The listing builds one solid part. Answer for the finished solid, in the listing's coordinates (mm). A direction names the side the tool comes from. Round coordinates to 2 decimals unless told otherwise and drop trailing zeros. Write each loop counter-clockwise with the first axis right and the second up, starting at its lowest first coordinate (ties: lowest second). Pieces come first, ordered by that corner, then holes. Notation, with made-up numbers: (-38, -10.5) - (19, -10.5) arc R32 cw to (19, 27.5) - close; hole circle Ø6 at (-4.75, 75.25). An arc over 180 degrees is marked (long way). Answer as CSV lines item,"result". Start each with the question number.
Item 1: A cutting plane is placed at C-C on y = 42. Determine the outline of the cut face in (x, z).
Item 2: Flat-ended cylindrical pins translate along their axes: pin 1 (1.5 mm diameter, centred on x = 35, z = 1.5, fed in from -Y); pin 2 (6 mm diameter, centred on x = 25.5, y = 20, fed in from -Z); pin 3 (1.5 mm diameter, centred on x = 36.5, z = 3, fed in from +Y). Find the tip coordinate at first contact, or state that the pin passes through.
Item 3: A cutting plane is placed at D-D on z = 4. State how many separate pieces and enclosed holes the cut face has, and give its area (3 significant figures).
Item 4: A cutting plane is placed at A-A on y = 104.5. Determine the outline of the cut face in (x, z), and give its area (3 significant figures).
Item 5: A cutting plane is placed at B-B on x = 12. Determine the outline of the cut face in (y, z), and give its area (3 significant figures).
Item 6: For a pull along X with two mould halves and no side action, classify faces 4 (the flat face through (0, 96, 2)), 5 (the flat face through (12, 195, 2)), 6 (the flat face through (25, -3, 2)) as pulls with the +X half, pulls with the -X half, needs draft (parallel to the pull), parting line crosses it, or undercut.
Item 7: Which of the six approach directions +Z, -Z, +X, -X, +Y, -Y give full straight-line access (tool end or side, diameter ignored) to faces 1 (the flat face through (45, -3, 2)), 2 (the flat face through (35, 190, 2)), 3 (the flat face through (60, 51, 3))?
Item 8: Straight lines are drawn through the part: line 1 along Y through (x, z) = (31.5, 0.8); line 2 along Y through (x, z) = (47, 2.05); line 3 along X through (y, z) = (151, 1.75). For each, find the intervals that lie inside material, in ascending order. Write a range as [from, to].
```python
from build123d import *

# Parameters (mm, degrees)
SKETCH_1_W          = 25
SKETCH_1_H          = 5
SKETCH_1_W_2        = 70
SKETCH_1_H_2        = 190
EXTRUDE_1_DEPTH     = 5
SKETCH_2_R          = 1.55
CUT_EXTRUDE_1_DEPTH = 5
SKETCH_3_W          = 50
SKETCH_3_H          = 72.5
CUT_EXTRUDE_2_DEPTH = 5
FILLET_1_R          = 10
FILLET_2_R          = 1


with BuildPart() as part:
    # 草图1 → 凸台-拉伸1 (new body)
    with BuildSketch(Plane.XY):
        with Locations((57.5, 192.5)):
            Rectangle(SKETCH_1_W, SKETCH_1_H)
        with Locations((35, 95)):
            Rectangle(SKETCH_1_W_2, SKETCH_1_H_2)
        with Locations((12.5, 192.5)):
            Rectangle(SKETCH_1_W, SKETCH_1_H)
        with Locations((57.5, -2.5)):
            Rectangle(SKETCH_1_W, SKETCH_1_H)
        with Locations((12.5, -2.5)):
            Rectangle(SKETCH_1_W, SKETCH_1_H)
    extrude(amount=EXTRUDE_1_DEPTH)

    # 草图2 → 切除-拉伸1 (cut)
    with BuildSketch(Plane.XY.offset(5)):
        with Locations((43.45, 0)):
            Circle(SKETCH_2_R)
        with Locations((26.55, 0)):
            Circle(SKETCH_2_R)
        with Locations((43.45, 190)):
            Circle(SKETCH_2_R)
        with Locations((26.55, 190)):
            Circle(SKETCH_2_R)
    extrude(amount=-CUT_EXTRUDE_1_DEPTH, mode=Mode.SUBTRACT)

    # 草图3 → 切除-拉伸2 (cut)
    with BuildSketch(Plane.XY.offset(5)):
        with Locations((35, 51.25)):
            Rectangle(SKETCH_3_W, SKETCH_3_H)
        with Locations((35, 138.75)):
            Rectangle(SKETCH_3_W, SKETCH_3_H)
    extrude(amount=-CUT_EXTRUDE_2_DEPTH, mode=Mode.SUBTRACT)

    # 圆角1
    fillet_1_edges = [part.edges().sort_by_distance(p)[0] for p in [
        (10, 15, 2.5),
        (10, 87.5, 2.5),
        (60, 87.5, 2.5),
        (60, 15, 2.5),
        (10, 102.5, 2.5),
        (10, 175, 2.5),
        (60, 175, 2.5),
        (60, 102.5, 2.5),
    ]]
    fillet(fillet_1_edges, radius=FILLET_1_R)

    # 圆角2
    fillet_2_edges = [part.edges().sort_by_distance(p)[0] for p in [
        (45, 195, 2.5),
        (70, 195, 2.5),
        (70, -5, 2.5),
        (0, -5, 2.5),
        (0, 195, 2.5),
        (25, 195, 2.5),
    ]]
    fillet(fillet_2_edges, radius=FILLET_2_R)


solid = part.part
```
Geometry says:
1,outline,"(0, 0) - (10, 0) - (10, 5) - (0, 5) - close; (60, 0) - (70, 0) - (70, 5) - (60, 5) - close"
2,pin 1,"stops at y = 0"
2,pin 2,"passes through"
2,pin 3,"stops at y = 190"
3,separate pieces,"1"
3,enclosed holes,"2"
3,area,"6,710 mm^2"
4,outline,"(0, 0) - (14, 0) - (14, 5) - (0, 5) - close; (56, 0) - (70, 0) - (70, 5) - (56, 5) - close"
4,area,"140 mm^2"
5,outline,"(-5, 0) - (19, 0) - (19, 5) - (-5, 5) - close; (83.5, 0) - (106.5, 0) - (106.5, 5) - (83.5, 5) - close; (171, 0) - (195, 0) - (195, 5) - (171, 5) - close"
5,area,"355 mm^2"
6,face 4,"pulls with the -X half"
6,face 5,"needs draft"
6,face 6,"undercut"
7,face 1,"+Z, -Z, -Y"
7,face 2,"+Z, -Z, +Y"
7,face 3,"+Z, -Z"
8,line 1,"y = [0, 15], [87.5, 102.5], [175, 190]"
8,line 2,"y = [-5, 15], [87.5, 102.5], [175, 195]"
8,line 3,"x = [0, 10], [60, 70]"
